from build123d import *

# Parameters (mm, degrees)
SKETCH1_R           = 15
SKETCH1_R_2         = 3
BOSS_EXTRUDE1_DEPTH = 5
SKETCH2_R           = 6
SKETCH2_R_2         = 4
BOSS_EXTRUDE2_DEPTH = 20


with BuildPart() as part:
    # Sketch1 → Boss-Extrude1 (new body)
    with BuildSketch(Plane(origin=(0, 0, 0), x_dir=(1, 0, 0), z_dir=(0, 1, 0))):
        Circle(SKETCH1_R)
        with Locations((0, 10)):
            Circle(SKETCH1_R_2, mode=Mode.SUBTRACT)
        with Locations((0, -10)):
            Circle(SKETCH1_R_2, mode=Mode.SUBTRACT)
    extrude(amount=BOSS_EXTRUDE1_DEPTH)

    # Sketch2 → Boss-Extrude2 (add)
    with BuildSketch(Plane(origin=(0, 5, 0), x_dir=(1, 0, 0), z_dir=(0, 1, 0))):
        Circle(SKETCH2_R)
        Circle(SKETCH2_R_2, mode=Mode.SUBTRACT)
    extrude(amount=BOSS_EXTRUDE2_DEPTH)


solid = part.part
The model under review builds one solid part; all positions refer to its coordinate system, in mm. A direction names the side the tool comes from. Coordinates: 2 decimals unless noted, no trailing zeros. Loops run counter-clockwise (first coordinate to the right, second up) from the corner with the lowest first, then second, coordinate; pieces in that order, holes last. Notation, with made-up numbers: (9.5, -34) -> (41.5, -34) arc R16 cw to (41.5, -13) -> close; hole circle Ø8 at (89.5, 29). An arc over 180 degrees is marked (long way). Use a Markdown table: item, result. Add a question column.
1. Draft analysis for pull direction X (two halves, no side actions). For faces 3 (the face through (6.5, 5, -0.2)), 4 (the face through (-6, 15, 0)), 5 (the face through (0, 2, 7)), state which applies: pulls with the +X half, pulls with the -X half, needs draft (parallel to the pull), parting line crosses it, or undercut.
2. To check wall thickness, follow line 1 (Z direction, x = 0, y = 3.8); line 2 (X direction, y = 13.5, z = 0); line 3 (Y direction, x = 7, z = 9). State the ranges of each line that lie inside material, in increasing order.
3. Clearance check with flat-ended pins moving along their axes: pin 1 Ø3 at (y, z) = (19, 6) entering from +X; pin 2 Ø10 at (y, z) = (12, 1.5) entering from -X; pin 3 Ø1.5 at (y, z) = (14, -6) entering from +X. State where each tip first meets the part, or that it passes through.
4. Add section D-D on y = 21.25. Write out the cut boundary in (x, z), plus the area to 3 significant figures.
5. Add section A-A on x = 0. Write out the cut boundary in (y, z).
6. Add section C-C on z = -10. Write out the cut boundary in (x, y).
7. Add section B-B on z = 0. Write out the cut boundary in (x, y), plus the area to 3 significant figures.
8. Machinability: for faces 1 (the face through (0, 5, 0)), 2 (the face through (-1.42, 25, 3.92)), which of the approach directions +Z, -Z, +X, -X, +Y, -Y give a long, thin tool a straight path to every point of the face, cutting with its end or side? Answer none if there is none.
Returned:
| question | item | result |
|---|---|---|
| 1 | face 3 | needs draft |
| 1 | face 4 | parting line crosses it |
| 1 | face 5 | undercut |
| 2 | line 1 | z = -15 to -13, -7 to 7, 13 to 15 |
| 2 | line 2 | x = -6 to -4, 4 to 6 |
| 2 | line 3 | y = 0 to 5 |
| 3 | pin 1 | stops at x = 3.97 |
| 3 | pin 2 | stops at x = -6 |
| 3 | pin 3 | stops at x = 2.9 |
| 4 | outline | circle Ø12 at (0, 0); hole circle Ø8 at (0, 0) |
| 4 | area | 62.8 mm² |
| 5 | outline | (0, -15) -> (5, -15) -> (5, -13) -> (0, -13) -> close; (0, -7) -> (5, -7) -> (5, -6) -> (25, -6) -> (25, -4) -> (5, -4) -> (5, 4) -> (25, 4) -> (25, 6) -> (5, 6) -> (5, 7) -> (0, 7) -> close; (0, 13) -> (5, 13) -> (5, 15) -> (0, 15) -> close |
| 6 | outline | (-11.18, 0) -> (-3, 0) -> (-3, 5) -> (-11.18, 5) -> close; (3, 0) -> (11.18, 0) -> (11.18, 5) -> (3, 5) -> close |
| 7 | outline | (-15, 0) -> (15, 0) -> (15, 5) -> (6, 5) -> (6, 25) -> (4, 25) -> (4, 5) -> (-4, 5) -> (-4, 25) -> (-6, 25) -> (-6, 5) -> (-15, 5) -> close |
| 7 | area | 230 mm² |
| 8 | face 1 | +Y |
| 8 | face 2 | +Z, -Z, +X, -X, +Y |
